Model file for the job. Use its own axes, mm. Give positions to 0.01 mm unless a question says otherwise; leave off trailing zeros.
```python
from build123d import *

# Parameters (mm, degrees)
BOSS_EXTRUDE1_DEPTH = 1.5875
FILLET1_R           = 1
SKETCH2_R           = 0.45
CUT_EXTRUDE1_DEPTH  = 71.728496069
SKETCH4_W           = 6.5
SKETCH4_H           = 6.5
BOSS_EXTRUDE2_DEPTH = 0.01
SKETCH5_OUTSIDE_W   = 130.286
SKETCH5_OUTSIDE_H   = 130.286
SKETCH5_OUTSIDE_W_2 = 99
SKETCH5_OUTSIDE_H_2 = 100
CUT_EXTRUDE3_DEPTH  = 71.728721226


with BuildPart() as part:
    # Sketch1 → Boss-Extrude1 (new body)
    with BuildSketch(Plane.XY):
        Polygon((40, 50), (-40, 50), (-40, 48), (-48, 48), (-48, 40), (-50, 40), (-50, -37.864895224), (-50, -40), (-48, -40), (-48, -48), (-40, -48), (-40, -50), (-37.864895224, -50), (40, -50), (40, -48), (48, -48), (48, -40), (50, -40), (50, 40), (48, 40), (48, 48), (40, 48), align=None)
    extrude(amount=BOSS_EXTRUDE1_DEPTH)

    # Fillet1
    fillet1_edges = [part.edges().sort_by_distance(p)[0] for p in [
        (-48, -40, 0.79375),
        (-48, 40, 0.79375),
        (-40, 48, 0.79375),
        (40, 48, 0.79375),
        (48, 40, 0.79375),
        (48, -40, 0.79375),
        (40, -48, 0.79375),
        (-40, -48, 0.79375),
    ]]
    fillet(fillet1_edges, radius=FILLET1_R)

    # Sketch2 → Cut-Extrude1 (cut, through all)
    with BuildSketch(Plane.XY.offset(1.5875)):
        with Locations((-35, 43.55)):
            Circle(SKETCH2_R)
        with Locations((-33, 43.55)):
            Circle(SKETCH2_R)
        with Locations((-31, 43.55)):
            Circle(SKETCH2_R)
        with Locations((-29, 43.55)):
            Circle(SKETCH2_R)
        with Locations((-27, 43.55)):
            Circle(SKETCH2_R)
        with Locations((-25, 43.55)):
            Circle(SKETCH2_R)
        with Locations((-23, 43.55)):
            Circle(SKETCH2_R)
        with Locations((-21, 43.55)):
            Circle(SKETCH2_R)
        with Locations((-19, 43.55)):
            Circle(SKETCH2_R)
        with Locations((-17, 43.55)):
            Circle(SKETCH2_R)
        with Locations((-15, 43.55)):
            Circle(SKETCH2_R)
        with Locations((-13, 43.55)):
            Circle(SKETCH2_R)
        with Locations((-11, 43.55)):
            Circle(SKETCH2_R)
        with Locations((-9, 43.55)):
            Circle(SKETCH2_R)
        with Locations((-7, 43.55)):
            Circle(SKETCH2_R)
        with Locations((-5, 43.55)):
            Circle(SKETCH2_R)
        with Locations((-3, 43.55)):
            Circle(SKETCH2_R)
        with Locations((-1, 43.55)):
            Circle(SKETCH2_R)
        with Locations((1, 43.55)):
            Circle(SKETCH2_R)
        with Locations((3, 43.55)):
            Circle(SKETCH2_R)
        with Locations((5, 43.55)):
            Circle(SKETCH2_R)
        with Locations((7, 43.55)):
            Circle(SKETCH2_R)
        with Locations((-33, 41.55)):
            Circle(SKETCH2_R)
        with Locations((-31, 41.55)):
            Circle(SKETCH2_R)
        with Locations((-29, 41.55)):
            Circle(SKETCH2_R)
        with Locations((-27, 41.55)):
            Circle(SKETCH2_R)
        with Locations((-25, 41.55)):
            Circle(SKETCH2_R)
        with Locations((-23, 41.55)):
            Circle(SKETCH2_R)
        with Locations((-21, 41.55)):
            Circle(SKETCH2_R)
        with Locations((-19, 41.55)):
            Circle(SKETCH2_R)
        with Locations((-17, 41.55)):
            Circle(SKETCH2_R)
        with Locations((-15, 41.55)):
            Circle(SKETCH2_R)
        with Locations((-13, 41.55)):
            Circle(SKETCH2_R)
        with Locations((-11, 41.55)):
            Circle(SKETCH2_R)
        with Locations((-9, 41.55)):
            Circle(SKETCH2_R)
        with Locations((-7, 41.55)):
            Circle(SKETCH2_R)
        with Locations((-5, 41.55)):
            Circle(SKETCH2_R)
        with Locations((-3, 41.55)):
            Circle(SKETCH2_R)
        with Locations((-1, 41.55)):
            Circle(SKETCH2_R)
        with Locations((1, 41.55)):
            Circle(SKETCH2_R)
        with Locations((3, 41.55)):
            Circle(SKETCH2_R)
        with Locations((5, 41.55)):
            Circle(SKETCH2_R)
        with Locations((7, 41.55)):
            Circle(SKETCH2_R)
        with Locations((-35, 41.55)):
            Circle(SKETCH2_R)
    extrude(amount=-CUT_EXTRUDE1_DEPTH, mode=Mode.SUBTRACT)

    # Sketch4 → Boss-Extrude2 (add)
    with BuildSketch(Plane.XY.offset(1.5875)):
        with Locations((-44.75, 44.75)):
            Rectangle(SKETCH4_W, SKETCH4_H)
        with Locations((-44.75, -44.75)):
            Rectangle(SKETCH4_W, SKETCH4_H)
        with Locations((44.75, -44.75)):
            Rectangle(SKETCH4_W, SKETCH4_H)
        with Locations((44.75, 44.75)):
            Rectangle(SKETCH4_W, SKETCH4_H)
    extrude(amount=BOSS_EXTRUDE2_DEPTH)

    # Sketch5 outside → Cut-Extrude3 (cut, through all)
    with BuildSketch(Plane(origin=(0, 0, 0), x_dir=(-1, 0, 0), z_dir=(0, 0, -1))):
        Rectangle(SKETCH5_OUTSIDE_W, SKETCH5_OUTSIDE_H)
        Rectangle(SKETCH5_OUTSIDE_W_2, SKETCH5_OUTSIDE_H_2, mode=Mode.SUBTRACT)
    extrude(amount=-CUT_EXTRUDE3_DEPTH, mode=Mode.SUBTRACT)


solid = part.part
```
1. Pin check, flat tips, straight feed: P1, Ø0.8, axis at y = -46, z = 0.5, coming from the +X side; P2, Ø0.5, axis at y = -44.5, z = 1, coming from the -X side; P3, Ø0.5, axis at x = 45, z = 0.5, coming from the +Y side. Stop position of each tip, or through.
Calculated:
P1: stops at x = 48
P2: stops at x = -48
P3: stops at y = 48
2. Probe probe 1 along Y at (x, z) = (-15, 0.8); probe 2 along Y at (x, z) = (-43, 1.15); probe 3 along Z at (x, y) = (17, -12). List the from-to ranges inside material, lowest first.
Calculated:
probe 1: y = -50 to 41.1, 42 to 43.1, 44 to 50
probe 2: y = -48 to 48
probe 3: z = 0 to 1.59
3. Slice it at A-A, the plane z = 1.3. State how many separate pieces and enclosed holes the cut face has, and give its area (3 significant figures).
Calculated:
separate pieces: 1
enclosed holes: 44
area: 9,750 mm2
